Input: part model. Units: mm. Frame: model coordinates. Coordinates: 2 decimals unless noted, no trailing zeros. Loops run counter-clockwise (first coordinate to the right, second up) from the corner with the lowest first, then second, coordinate; pieces in that order, holes last. Notation, with made-up numbers: (-3, 79) - (18, 79) arc R7 ccw to (18, 87) - close; hole circle Ø9 at (12, -2.75). An arc over 180 degrees is marked (long way). Write item = value, one per line. Start each with the question number.
from build123d import *

# Parameters (mm, degrees)
SKETCH1_W               = 75.050000014
SKETCH1_H               = 457.2
BOSS_EXTRUDE1_DEPTH     = 3.175
SKETCH8_W               = 3.175
SKETCH8_H               = 19.05
CUT_EXTRUDE2_DEPTH      = 232.681173708
CRVPATTERN1_START       = -31.175
CRVPATTERN1_OUTLINE_W   = 19.05
CRVPATTERN1_OUTLINE_H   = 3.175
CRVPATTERN1_DEPTH       = 3.175
CRVPATTERN1_START_2     = 28
CRVPATTERN1_2_OUTLINE_W = 19.05
CRVPATTERN1_2_OUTLINE_H = 3.175
CRVPATTERN1_2_DEPTH     = 3.175
SKETCH10_R              = 6.731
CUT_EXTRUDE3_DEPTH      = 232.681173708
F_10_CLEARANCE_HOLE1_D  = 5.1054


# Read off the part's stored shape, not the designer's step: CrvPattern1
with BuildPart() as part:
    # Sketch1 → Boss-Extrude1 (new body)
    with BuildSketch(Plane.XY):
        Rectangle(SKETCH1_W, SKETCH1_H)
    extrude(amount=BOSS_EXTRUDE1_DEPTH)

    # Sketch8 → Cut-Extrude2 (cut, through all)
    with BuildSketch(Plane(origin=(0, 0, 0), x_dir=(-1, 0, 0), z_dir=(0, 0, -1))):
        with Locations((-29.5875, 206.375)):
            Rectangle(SKETCH8_W, SKETCH8_H)
        with Locations((29.5875, 206.375)):
            Rectangle(SKETCH8_W, SKETCH8_H)
    extrude(amount=-CUT_EXTRUDE2_DEPTH, mode=Mode.SUBTRACT)

    # CrvPattern1 outline → CrvPattern1 (cut)
    with BuildSketch(Plane.YZ.offset(CRVPATTERN1_START)):
        with Locations((147.410714286, 1.5875)):
            Rectangle(CRVPATTERN1_OUTLINE_W, CRVPATTERN1_OUTLINE_H)
        with Locations((88.446428571, 1.5875)):
            Rectangle(CRVPATTERN1_OUTLINE_W, CRVPATTERN1_OUTLINE_H)
        with Locations((29.482142857, 1.5875)):
            Rectangle(CRVPATTERN1_OUTLINE_W, CRVPATTERN1_OUTLINE_H)
        with Locations((-29.482142857, 1.5875)):
            Rectangle(CRVPATTERN1_OUTLINE_W, CRVPATTERN1_OUTLINE_H)
        with Locations((-88.446428571, 1.5875)):
            Rectangle(CRVPATTERN1_OUTLINE_W, CRVPATTERN1_OUTLINE_H)
        with Locations((-147.410714286, 1.5875)):
            Rectangle(CRVPATTERN1_OUTLINE_W, CRVPATTERN1_OUTLINE_H)
        with Locations((-206.375, 1.5875)):
            Rectangle(CRVPATTERN1_OUTLINE_W, CRVPATTERN1_OUTLINE_H)
    extrude(amount=CRVPATTERN1_DEPTH, mode=Mode.SUBTRACT)

    # CrvPattern1 2 outline → CrvPattern1 2 (cut)
    with BuildSketch(Plane.YZ.offset(CRVPATTERN1_START_2)):
        with Locations((147.410714286, 1.5875)):
            Rectangle(CRVPATTERN1_2_OUTLINE_W, CRVPATTERN1_2_OUTLINE_H)
        with Locations((88.446428571, 1.5875)):
            Rectangle(CRVPATTERN1_2_OUTLINE_W, CRVPATTERN1_2_OUTLINE_H)
        with Locations((29.482142857, 1.5875)):
            Rectangle(CRVPATTERN1_2_OUTLINE_W, CRVPATTERN1_2_OUTLINE_H)
        with Locations((-29.482142857, 1.5875)):
            Rectangle(CRVPATTERN1_2_OUTLINE_W, CRVPATTERN1_2_OUTLINE_H)
        with Locations((-88.446428571, 1.5875)):
            Rectangle(CRVPATTERN1_2_OUTLINE_W, CRVPATTERN1_2_OUTLINE_H)
        with Locations((-147.410714286, 1.5875)):
            Rectangle(CRVPATTERN1_2_OUTLINE_W, CRVPATTERN1_2_OUTLINE_H)
        with Locations((-206.375, 1.5875)):
            Rectangle(CRVPATTERN1_2_OUTLINE_W, CRVPATTERN1_2_OUTLINE_H)
    extrude(amount=CRVPATTERN1_2_DEPTH, mode=Mode.SUBTRACT)

    # Sketch10 → Cut-Extrude3 (cut, through all)
    with BuildSketch(Plane(origin=(0, 0, 0), x_dir=(-1, 0, 0), z_dir=(0, 0, -1))):
        with Locations((0, -209.55)):
            Circle(SKETCH10_R)
    extrude(amount=-CUT_EXTRUDE3_DEPTH, mode=Mode.SUBTRACT)

    # #10 Clearance Hole1 (through all)
    with Locations(Plane(origin=(0, 0, 0), x_dir=(-1, 0, 0), z_dir=(0, 0, -1))):
        with Locations((18.602, -214.63), (18.602, -204.47), (-18.602, -214.63), (-18.602, -280.67)):
            Hole(F_10_CLEARANCE_HOLE1_D / 2)


solid = part.part
Item 1: Cut plane A-A on x = 0. Return loops of the section in (y, z) (3 decimals).
Item 2: Pull-direction query (Y, two-part tool) for faces 1 (the cylindrical face through (1.46, -216.12, 1.57)), 2 (the flat face through (-1, 3, 3.175)); classes: pulls with the +Y half, pulls with the -Y half, needs draft (parallel to the pull), parting line crosses it, or undercut.
Item 3: Ray query, line 1 (X direction, y = -151, z = 2.85) (3 decimals); line 2 (Y direction, x = 0, z = 2.55); line 3 (Y direction, x = 19, z = 1.3). Return the intervals inside material, ascending.
Item 4: Cut plane B-B on z = 1.05. State how many separate pieces and enclosed holes the cut face has, plus the area to 3 significant figures.
Recorded:
q1.outline = (-228.6, 0) - (-216.281, 0) - (-216.281, 3.175) - (-228.6, 3.175) - close; (-202.819, 0) - (228.6, 0) - (228.6, 3.175) - (-202.819, 3.175) - close
q2.face_1 = undercut
q2.face_2 = needs draft
q3.line_1 = -37.525 to -31.175, -28 to 28, 31.175 to 37.525
q3.line_2 = -228.6 to -216.28, -202.82 to 228.6
q3.line_3 = -228.6 to -217.15, -212.11 to 228.6
q4.separate_pieces = 1
q4.enclosed_holes = 20
q4.area = 33,100 mm²
